Can you work these out from the drawing? Everything is in mm from the part's minimum corner. Coordinates: 2 decimals unless noted, no trailing zeros. Loops run counter-clockwise (first coordinate to the right, second up) from the corner with the lowest first, then second, coordinate; pieces in that order, holes last. Notation, with made-up numbers: (7, 33.25) -> (66, 33.25) arc R16 cw to (66, 43.25) -> close; hole circle Ø6 at (17, 16). An arc over 180 degrees is marked (long way). Put each result on its own line as item: value. Start each with the question number.
Item 1: If we section it at A-A on y = 27.88: Please give me the cut outline in (x, z) (3 decimals).
Item 2: If we section it at D-D on x = 11.5: Please give me the cut outline in (y, z).
Item 3: If we section it at B-B on x = 18: Please give me the cut outline in (y, z), plus the area to 3 significant figures.
Item 4: We'd pull the mould along Y, two halves only. Please class the marked faces 1, 2 and 3: pulls with the +Y half, pulls with the -Y half, needs draft (parallel to the pull), parting line crosses it, or undercut.
Item 5: Please list where these lines run through material, in increasing order: L1, parallel to X at y = 28, z = 2.75 (1 decimal); L2, parallel to Y at x = 16.75, z = 1.5; L3, parallel to X at y = 33, z = 7 (1 decimal). Write a range as from..to.
Item 6: If we section it at C-C on z = 6: Please give me the cut outline in (x, y) (1 decimal).
Item 7: Will these pins go through, and if not, where does the flat tip stop? P1, Ø3.5, axis at x = 4.885, y = 27.88, coming from the +Z side; P2, Ø1.5, axis at y = 35, z = 2.5, coming from the -X side.
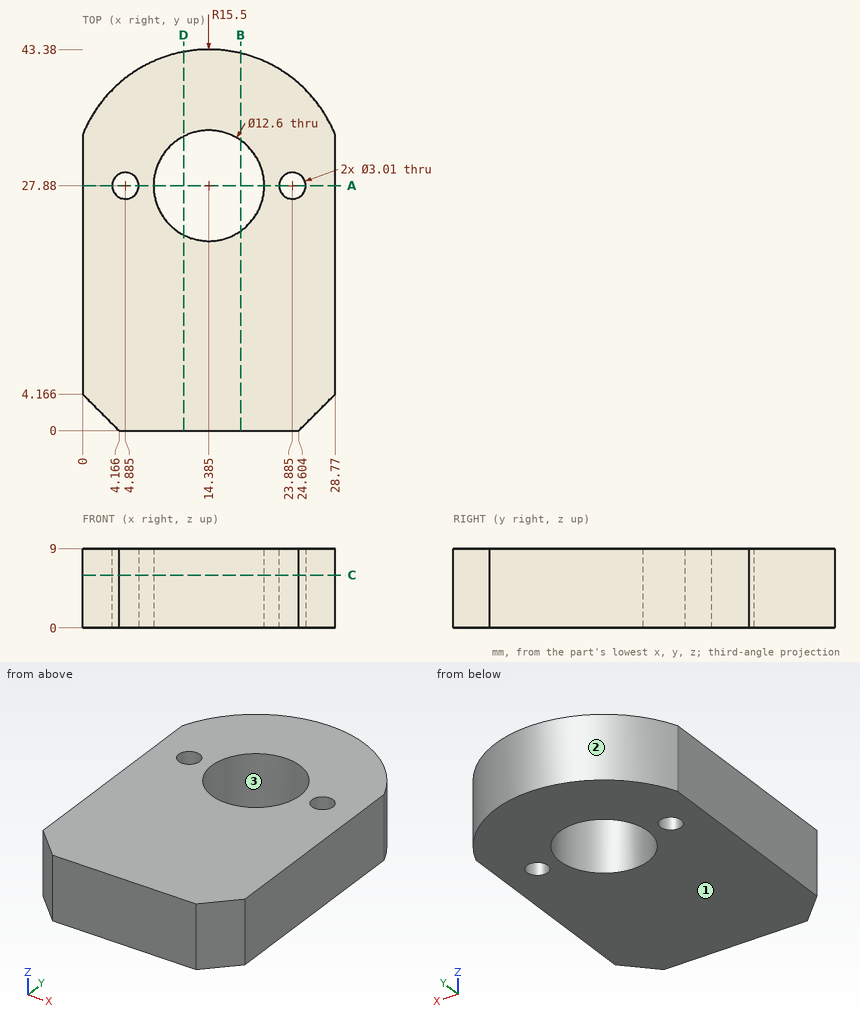
Solutions:
1. outline: (0, 0) -> (3.38, 0) -> (3.38, 9) -> (0, 9) -> close; (6.39, 0) -> (8.085, 0) -> (8.085, 9) -> (6.39, 9) -> close; (20.685, 0) -> (22.38, 0) -> (22.38, 9) -> (20.685, 9) -> close; (25.39, 0) -> (28.77, 0) -> (28.77, 9) -> (25.39, 9) -> close
2. outline: (0, 0) -> (22.28, 0) -> (22.28, 9) -> (0, 9) -> close; (33.48, 0) -> (43.11, 0) -> (43.11, 9) -> (33.48, 9) -> close
3. outline: (0, 0) -> (22.72, 0) -> (22.72, 9) -> (0, 9) -> close; (33.04, 0) -> (42.95, 0) -> (42.95, 9) -> (33.04, 9) -> close
3. area: 294 mm^2
4. face 1: needs draft
4. face 2: pulls with the +Y half
4. face 3: undercut
5. L1: 0..3.4, 6.4..8.1, 20.7..22.4, 25.4..28.8
5. L2: 0..22.04, 33.72..43.2
5. L3: 0..10.7, 18.1..28.8
6. outline: (0, 4.2) -> (4.2, 0) -> (24.6, 0) -> (28.8, 4.2) -> (28.8, 33.7) arc R15.5 ccw to (0, 33.7) -> close; hole circle Ø3 at (4.9, 27.9); hole circle Ø12.6 at (14.4, 27.9); hole circle Ø3 at (23.9, 27.9)
7. P1: z = 9
7. P2: x = 0.25
